Part model, mm, in its own coordinate system. A direction names the side the tool comes from. Round coordinates to 2 decimals unless told otherwise and drop trailing zeros. Order: outer loops, then holes, each group sorted by start corner. A loop starts at its lowest first (then second) coordinate and runs counter-clockwise, first axis right, second up. Notation, with made-up numbers: (71.5, 53.25) - (78.5, 53.25) arc R8 cw to (78.5, 57.25) - close; hole circle Ø10 at (-15.5, -34.75). An arc over 180 degrees is marked (long way). Answer as a JSON object with one key per item and string values.
```python
from build123d import *

# Parameters (mm, degrees)
SKIZZE2_R                       = 1
SCHNITT_LINEAR_AUSTRAGEN1_DEPTH = 4
FASE1_SIZE                      = 0.25


with BuildPart() as part:
    # Skizze1 → Rotation1 (revolve)
    with BuildSketch(Plane(origin=(0, 0, 0), x_dir=(0, 0, -1), z_dir=(1, 0, 0))):
        Polygon((0, 1), (10, 1), (10, 3), (-10, 3), (-10, 1.6), (-26, 1.6), (-26, 0), (0, 0), align=None)
    revolve(axis=Axis((0, 0, 0), (0, 0, 1)))

    # Skizze2 → Schnitt-Linear austragen1 (cut, through all)
    with BuildSketch(Plane(origin=(0, 0, 0), x_dir=(1, 0, 0), z_dir=(0, 1, 0))):
        with Locations((0, 2)):
            Circle(SKIZZE2_R)
    extrude(amount=SCHNITT_LINEAR_AUSTRAGEN1_DEPTH, mode=Mode.SUBTRACT)

    # Fase1
    fase1_edges = [part.edges().sort_by_distance(p)[0] for p in [
        (0, -3, -10),
        (0, -3, 10),
        (0, -1.6, 26),
    ]]
    chamfer(fase1_edges, length=FASE1_SIZE)


solid = part.part
```
Item 1: Tool access for faces 5 (the cylindrical face through (0.97, -1.27, 17.99)), 6 (the flat face through (0, 0, 0)): list every direction of +Z, -Z, +X, -X, +Y, -Y with a clear straight run to the whole face (end or side of a thin tool).
Taken from the geometry:
{"face 5": "+Z", "face 6": "-Z"}
Item 2: Two-plate mould, pull along Z, no slides. Class faces 1 (the flat face through (1.2, 0, -10)), 2 (the flat face through (0, 0, 26)), 3 (the cylindrical face through (1.8, -2.4, 0.1)), 4 (the cylindrical face through (-1, 2, -2)): pulls with the +Z half, pulls with the -Z half, needs draft (parallel to the pull), parting line crosses it, or undercut.
Taken from the geometry:
{"face 1": "pulls with the -Z half", "face 2": "pulls with the +Z half", "face 3": "needs draft", "face 4": "undercut"}
Item 3: Cut at A-A (x = 0). Write the cut outline in (y, z).
Taken from the geometry:
{"outline": "(-3, -9.75) - (-2.75, -10) - (-1, -10) - (-1, 0) - (1, 0) - (1, -1) - (3, -1) - (3, 9.75) - (2.75, 10) - (1.6, 10) - (1.6, 25.75) - (1.35, 26) - (-1.35, 26) - (-1.6, 25.75) - (-1.6, 10) - (-2.75, 10) - (-3, 9.75) - close; (1, -10) - (2.75, -10) - (3, -9.75) - (3, -3) - (1, -3) - close"}
Item 4: Cut at B-B (z = -4). Write the cut outline in (x, y).
Taken from the geometry:
{"outline": "circle Ø6 at (0, 0); hole circle Ø2 at (0, 0)"}
Item 5: Cut at D-D (z = 5.5). Write the cut outline in (x, y).
Taken from the geometry:
{"outline": "circle Ø6 at (0, 0)"}
Item 6: Drop flat-ended pins along their axis: P1, Ø1.5, axis at x = 0, z = 21.5, coming from the -Y side; P2, Ø1.5, axis at x = -2, z = 1.5, coming from the -Y side; P3, Ø2, axis at y = -0.5, z = 18, coming from the -X side. Give the stop position or say it passes through.
Taken from the geometry:
{"P1": "y = -1.6", "P2": "y = -2.73", "P3": "x = -1.6"}
Item 7: Cut at C-C (z = 23). Write the cut outline in (x, y).
Taken from the geometry:
{"outline": "circle Ø3.2 at (0, 0)"}
Item 8: Probe L1, parallel to Z at x = 0, y = 2; L2, parallel to Y at x = 0, z = -5.5. List the from-to ranges inside material, lowest first. Write a range as from..to.
Taken from the geometry:
{"L1": "-10..-3, -1..10", "L2": "-3..-1, 1..3"}
